Can you work these out from the model? Positions are in its coordinate system, mm. Face numbers are marked on the shaded views. A direction names the side the tool comes from. Round coordinates to 2 decimals unless told otherwise and drop trailing zeros. Write each loop counter-clockwise with the first axis right and the second up, starting at its lowest first coordinate (ties: lowest second). Pieces come first, ordered by that corner, then holes. Notation, with made-up numbers: M 75.5,3.5 L 88.5,3.5 A23 ccw 88.5,22.5 Z; hole C 1.5,85.25 d7. An arc over 180 degrees is marked long. Answer as a JSON object with one key per item and string values. Group by question number.
1) Suppose I cut it at D-D, the plane x = 6.2. Write out the boundary of the cut face in (y, z).
2) Suppose I cut it at A-A, the plane x = 0. Write out the boundary of the cut face in (y, z), and give its area (3 significant figures).
3) Suppose I cut it at C-C, the plane z = 1. Write out the boundary of the cut face in (x, y), and give its area (3 significant figures).
4) Please list where these lines run through material, in increasing order: L1, parallel to Y at x = 6.2, z = 1.2; L2, parallel to Y at x = -1.25, z = -2; L3, parallel to Z at x = -6, y = 6.25. Write a range as [from, to].
5) If we mould it in two halves opening along Y, with no side actions, what happens to the marked faces 3, 4 and 5? For each: +Y half, -Y half, draft (parallel to the pull), parting line (faces both ways), or undercut.
6) I'm going to push flat-ended pins straight in: pin 1 Ø2 at (y, z) = (1, -2) entering from -X; pin 2 Ø1.5 at (x, y) = (-3.5, 5) entering from -Z; pin 3 Ø1.6 at (x, y) = (6.2, 0) entering from -Z; pin 4 Ø2.5 at (x, y) = (-6.2, 0) entering from +Z. Where does each tip first touch, or does it pass through?
7) On a 3-axis mill with a long thin cutter (end or side, diameter ignored), from which of +Z, -Z, +X, -X, +Y, -Y can I reach the whole of each face in a straight line? I mean the marked faces 1 and 2. Say none if no direction works.
from build123d import *

# Parameters (mm, degrees)
SKETCH1_R                = 9
SKETCH1_R_2              = 3.4
SKETCH1_R_3              = 1
BOSS_EXTRUDE1_DEPTH      = 2
BOSS_EXTRUDE2_DEPTH      = 5.6
BOSS_EXTRUDE2_DEPTH_BACK = 2.2
SKETCH2_R                = 3.6
SKETCH2_R_2              = 1.4
SKETCH3_R                = 2.75
CUT_EXTRUDE1_DEPTH       = 5.6


with BuildPart() as part:
    # Sketch1 → Boss-Extrude1 (new body)
    with BuildSketch(Plane.XY):
        Circle(SKETCH1_R)
        Circle(SKETCH1_R_2, mode=Mode.SUBTRACT)
        with Locations((0, 6.2)):
            Circle(SKETCH1_R_3, mode=Mode.SUBTRACT)
        with Locations((6.2, 0)):
            Circle(SKETCH1_R_3, mode=Mode.SUBTRACT)
        with Locations((0, -6.2)):
            Circle(SKETCH1_R_3, mode=Mode.SUBTRACT)
        with Locations((-6.2, 0)):
            Circle(SKETCH1_R_3, mode=Mode.SUBTRACT)
    extrude(amount=BOSS_EXTRUDE1_DEPTH)

    # Sketch2 → Boss-Extrude2 (add, two sides: drawn at the far end of the back side and taken through both)
    with BuildSketch(Plane(origin=(0, 0, 0), x_dir=(-1, 0, 0), z_dir=(0, 0, -1)).offset(-BOSS_EXTRUDE2_DEPTH_BACK)):
        Circle(SKETCH2_R)
        Circle(SKETCH2_R_2, mode=Mode.SUBTRACT)
    extrude(amount=BOSS_EXTRUDE2_DEPTH + BOSS_EXTRUDE2_DEPTH_BACK)

    # Sketch3 → Cut-Extrude1 (cut)
    with BuildSketch(Plane(origin=(0, 0, -5.6), x_dir=(-1, 0, 0), z_dir=(0, 0, -1))):
        Circle(SKETCH3_R)
    extrude(amount=-CUT_EXTRUDE1_DEPTH, mode=Mode.SUBTRACT)


solid = part.part
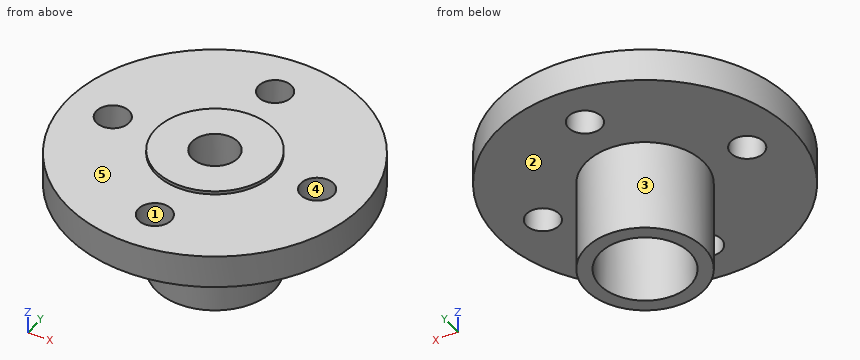
Results:
{
 "1": {"outline": "M -6.52,0 L -1,0 L -1,2 L -6.52,2 Z; M 1,0 L 6.52,0 L 6.52,2 L 1,2 Z"},
 "2": {"outline": "M -9,0 L -7.2,0 L -7.2,2 L -9,2 Z; M -5.2,0 L -3.6,0 L -3.6,-5.6 L -2.75,-5.6 L -2.75,0 L -1.4,0 L -1.4,2.2 L -3.6,2.2 L -3.6,2 L -5.2,2 Z; M 1.4,0 L 2.75,0 L 2.75,-5.6 L 3.6,-5.6 L 3.6,0 L 5.2,0 L 5.2,2 L 3.6,2 L 3.6,2.2 L 1.4,2.2 Z; M 7.2,0 L 9,0 L 9,2 L 7.2,2 Z", "area": "32.8 mm^2"},
 "3": {"outline": "C 0,0 d18; hole C -6.2,0 d2; hole C 0,0 d2.8; hole C 0,-6.2 d2; hole C 0,6.2 d2; hole C 6.2,0 d2", "area": "236 mm^2"},
 "4": {"L1": "[-6.52, -1], [1, 6.52]", "L2": "[-3.38, -2.45], [2.45, 3.38]", "L3": "[0, 2]"},
 "5": {"face 3": "parting line", "face 4": "undercut", "face 5": "draft"},
 "6": {"pin 1": "x = -3.6", "pin 2": "z = 0", "pin 3": "through", "pin 4": "z = 2"},
 "7": {"face 1": "+Z, -Z", "face 2": "-Z"}
}
